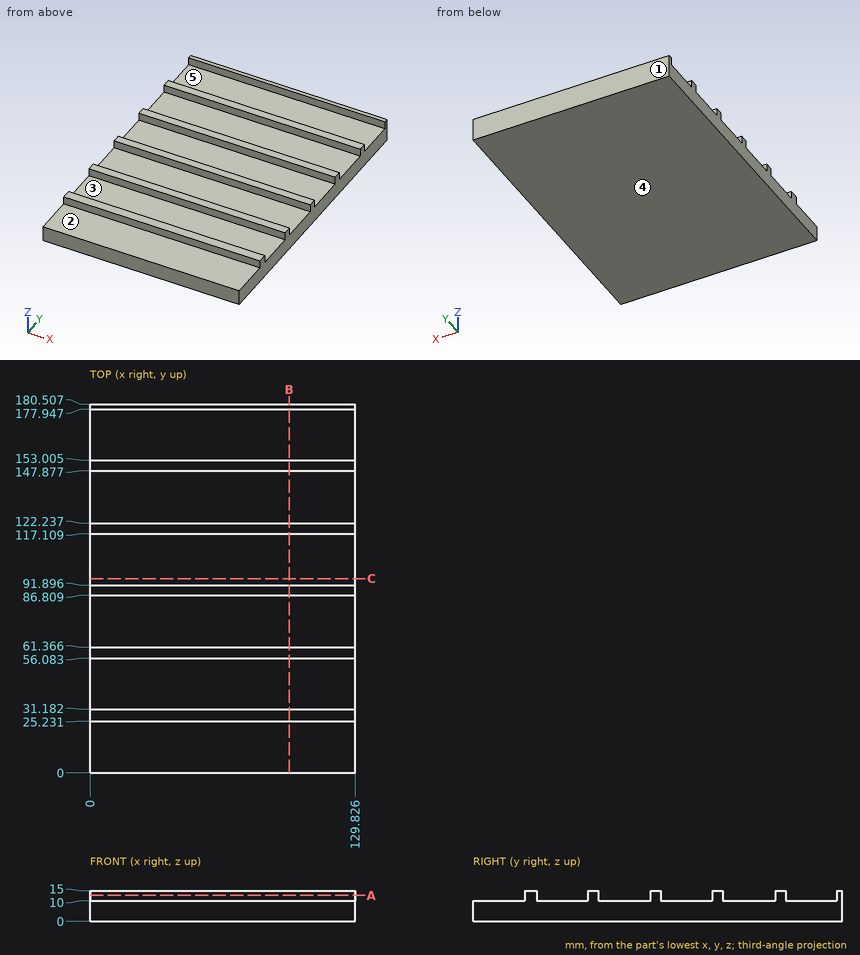
The figure shows three views and two pictorial views of one solid part (mm, origin at its lowest corner). Answer the questions. A direction names the side the tool comes from. Give positions to 0.01 mm unless a question says otherwise; leave off trailing zeros. Order: outer loops, then holes, each group sorted by start corner. A loop starts at its lowest first (then second) coordinate and runs counter-clockwise, first axis right, second up. Notation, with made-up numbers: (33, 53.5) -> (91, 53.5) arc R17 cw to (91, 72.5) -> close; hole circle Ø3 at (56.25, 9.25). An arc over 180 degrees is marked (long way). Write each question's results on one line, items separated by ' | '.
Q1. Straight lines are drawn through the part: probe 1 along Y at (x, z) = (15, 10.25) (1 decimal); probe 2 along Z at (x, y) = (104.5, 24). For each, find the intervals that lie inside material, in ascending order. Write a range as from..to.
Checked values:
probe 1: y = 25.2..31.2, 56.1..61.4, 86.8..91.9, 117.1..122.2, 147.9..153, 177.9..180.5 | probe 2: z = 0..10
Q2. Which of the six approach directions +Z, -Z, +X, -X, +Y, -Y give full straight-line access (tool end or side, diameter ignored) to the marked faces 4 and 5?
Checked values:
face 4: -Z, +X, -X, +Y, -Y | face 5: +Z, +X, -X
Q3. The part is cut by section B-B, the plane x = 97.5. Give the vertices of the cut face in (y, z) (1 decimal), and give its area (3 significant figures).
Checked values:
outline: (0, 0) -> (180.5, 0) -> (180.5, 15) -> (177.9, 15) -> (177.9, 10) -> (153, 10) -> (153, 15) -> (147.9, 15) -> (147.9, 10) -> (122.2, 10) -> (122.2, 15) -> (117.1, 15) -> (117.1, 10) -> (91.9, 10) -> (91.9, 15) -> (86.8, 15) -> (86.8, 10) -> (61.4, 10) -> (61.4, 15) -> (56.1, 15) -> (56.1, 10) -> (31.2, 10) -> (31.2, 15) -> (25.2, 15) -> (25.2, 10) -> (0, 10) -> close | area: 1,950 mm^2
Q4. The part is cut by section C-C, the plane y = 95. Give the vertices of the cut face in (x, z).
Checked values:
outline: (0, 0) -> (129.83, 0) -> (129.83, 10) -> (0, 10) -> close
Q5. The part is cut by section A-A, the plane z = 12.75. Give the vertices of the cut face in (x, y) (1 decimal).
Checked values:
outline: (0, 25.2) -> (129.8, 25.2) -> (129.8, 31.2) -> (0, 31.2) -> close; (0, 56.1) -> (129.8, 56.1) -> (129.8, 61.4) -> (0, 61.4) -> close; (0, 86.8) -> (129.8, 86.8) -> (129.8, 91.9) -> (0, 91.9) -> close; (0, 117.1) -> (129.8, 117.1) -> (129.8, 122.2) -> (0, 122.2) -> close; (0, 147.9) -> (129.8, 147.9) -> (129.8, 153) -> (0, 153) -> close; (0, 177.9) -> (129.8, 177.9) -> (129.8, 180.5) -> (0, 180.5) -> close
Q6. Each of these flat-tipped pins is pushed along its axis until it touches: P1, Ø7.5, axis at x = 96.5, y = 140.5, coming from the +Z side; P2, Ø4, axis at x = 41.5, z = 13, coming from the -Y side. Where does it stop, or does it pass through?
Checked values:
P1: stops at z = 10 | P2: stops at y = 25.23
Q7. Determine the mould class of the marked faces 1, 2 and 3 for opening direction Y: pulls with the +Y half, pulls with the -Y half, needs draft (parallel to the pull), parting line crosses it, or undercut.
Checked values:
face 1: pulls with the +Y half | face 2: needs draft | face 3: undercut
